Autodesk Inventor part; units mm, degrees
ref_plane "YZ Plane" through (0, 0, 0) normal (1, 0, 0) x (0, 1, 0)
ref_plane "XZ Plane" through (0, 0, 0) normal (0, 1, 0) x (-1, 0, 0)
ref_plane "XY Plane" through (0, 0, 0) normal (0, 0, 1) x (1, 0, 0)
sketch "Skizze4" plane through (0, 0, 0) normal (0, 0, 1) x (1, 0, 0)
  line L0 (0, 0) -> (200, 0)
  line L1 (200, 0) -> (200, 3)
  line L2 (200, 3) -> (0, 3)
  line L3 (0, 3) -> (0, 0)
  dimension "d12" = 200
  dimension "d13" = 3
extrude "Extrusion4" add sketch "Skizze4" along normal blind 3
sketch "Skizze5" plane through (0, 0, 3) normal (0, 0, 1) x (1, 0, 0)
  line L0 (47, 5) -> (50, 5)
  line L1 (50, 5) -> (50, -2)
  line L2 (50, -2) -> (47, -2)
  line L3 (47, -2) -> (47, 5)
  line L4 (200, 0) -> (200, 3)
  line L5 (0, 3) -> (0, 0)
  line L6 (200, 3) -> (0, 3)
  line L7 (0, 0) -> (200, 0)
  dimension "d16" = 150
  dimension "d17" = 47
  dimension "d18" = 2
  dimension "d19" = 2
extrude "Extrusion5" add sketch "Skizze5" along normal blind 2 and the other way blind 5 contours L0 L1 L6 L3 | L6 L1 L7 L3 | L7 L1 L2 L3
properties part number "MiddleStick"
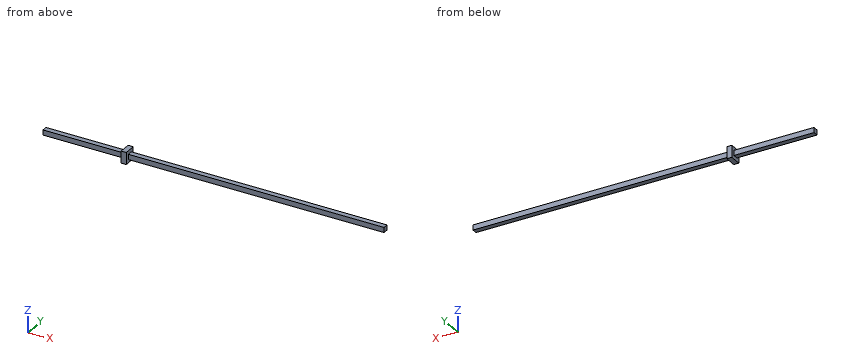
Read the model definition and answer for the solid it produces. Units are mm, in the model's axes. Give positions to 0.01 mm unless a question says otherwise; leave off trailing zeros. Loops run counter-clockwise (first coordinate to the right, second up) from the corner with the lowest first, then second, coordinate; pieces in that order, holes last. Notation, with made-up numbers: (-16.75, 18.5) - (4.25, 18.5) arc R23 ccw to (4.25, 42.5) - close; hole circle Ø1 at (82.25, 17.5). An arc over 180 degrees is marked (long way). Answer as CSV lines item,"result". Start each with the question number.
1) Each of these flat-tipped pins is pushed along its axis until it touches: pin 1 Ø3 at (x, y) = (168.5, -1) entering from -Z; pin 2 Ø3.5 at (x, z) = (31.5, 1) entering from +Y; pin 3 Ø1 at (x, y) = (80.5, 1.5) entering from +Z. Where does it stop, or does it pass through?
2) Find section A-A (x = 102.5). Write down the section's boundary in (y, z).
3) Straight lines are drawn through the part: L1, parallel to Y at x = 36, z = 1; L2, parallel to X at y = -1.5, z = 0. For each, find the intervals that lie inside material, in ascending order. Write a range as from..to.
Findings below:
1,pin 1,"z = 0"
1,pin 2,"y = 3"
1,pin 3,"z = 3"
2,outline,"(0, 0) - (3, 0) - (3, 3) - (0, 3) - close"
3,L1,"0..3"
3,L2,"47..50"
